Work out the finished part from the listing and answer in its coordinate system (mm). A direction names the side the tool comes from. Round coordinates to 2 decimals unless told otherwise and drop trailing zeros. Order: outer loops, then holes, each group sorted by start corner. A loop starts at its lowest first (then second) coordinate and runs counter-clockwise, first axis right, second up. Notation, with made-up numbers: (33.25, 0.5) - (48.25, 0.5) arc R20 ccw to (48.25, 5.5) - close; hole circle Ø9 at (47, 19.25). An arc over 180 degrees is marked (long way). Answer in a Markdown table with one row per item.
from build123d import *

# Parameters (mm, degrees)
BOSS_EXTRUDE1_DEPTH           = 2
CSK_FOR_M3_SFHCS1_D           = 3
CSK_FOR_M3_SFHCS1_DEPTH       = 9.5
CSK_FOR_M3_SFHCS1_CSINK_D     = 5.6
CSK_FOR_M3_SFHCS1_CSINK_ANGLE = 90
CSK_FOR_M3_SFHCS1_TIP         = 0.901290929
SKETCH6_R                     = 1.05
CUT_EXTRUDE1_DEPTH            = 6
SKETCH7_R                     = 1.05
CUT_EXTRUDE2_DEPTH            = 6
SKETCH8_R                     = 1.05
CUT_EXTRUDE3_DEPTH            = 6
M2_5X0_45_TAPPED_HOLE1_D      = 2.05
M2_5X0_45_TAPPED_HOLE1_DEPTH  = 6.35
M2_5X0_45_TAPPED_HOLE1_TIP    = 0.615882135
TAP_DRILL_FOR_M3X0_5_TAP1_D   = 2.5


with BuildPart() as part:
    # Sketch1 → Boss-Extrude1 (new, symmetric)
    with BuildSketch(Plane(origin=(0, 0, 0), x_dir=(1, 0, 0), z_dir=(0, 1, 0))):
        with BuildLine():
            Line((-48.836461788, 72), (48.836461788, 72))
            ThreePointArc((48.836461788, 72), (0, -87), (-48.836461788, 72))
        make_face()
        with BuildLine():
            Line((-46.314144708, 64), (46.314144708, 64))
            ThreePointArc((46.314144708, 64), (0, -79), (-46.314144708, 64))
        make_face(mode=Mode.SUBTRACT)
    extrude(amount=BOSS_EXTRUDE1_DEPTH, both=True)

    # CSK for M3 SFHCS1
    with Locations(Plane(origin=(-37.681211478, 2, 73.953541508), x_dir=(0, 0, 1), z_dir=(0, 1, 0))):
        with Locations((0, 0), (-141.953541508, -1.578606827), (-141.953541508, 76.941029783), (0, 75.362422956)):
            CounterSinkHole(CSK_FOR_M3_SFHCS1_D / 2, CSK_FOR_M3_SFHCS1_CSINK_D / 2, depth=CSK_FOR_M3_SFHCS1_DEPTH, counter_sink_angle=CSK_FOR_M3_SFHCS1_CSINK_ANGLE)
            with Locations((0, 0, -(CSK_FOR_M3_SFHCS1_DEPTH + CSK_FOR_M3_SFHCS1_TIP / 2))):  # 118° drill point
                Cone(0, CSK_FOR_M3_SFHCS1_D / 2, CSK_FOR_M3_SFHCS1_TIP, mode=Mode.SUBTRACT)

    # Sketch6 → Cut-Extrude1 (cut)
    with BuildSketch(Plane(origin=(75.344210129, 0, -43.5), x_dir=(-0.49999999999999784, 0, -0.86602540378444), z_dir=(0.86602540378444, 0, -0.49999999999999784))):
        Circle(SKETCH6_R)
    cut_extrude1 = extrude(amount=-CUT_EXTRUDE1_DEPTH, mode=Mode.SUBTRACT)

    # Sketch7 → Cut-Extrude2 (cut)
    with BuildSketch(Plane(origin=(75.344210129, 0, 43.5), x_dir=(0.5000000000000047, 0, -0.866025403784436), z_dir=(0.866025403784436, 0, 0.5000000000000047))):
        Circle(SKETCH7_R)
    cut_extrude2 = extrude(amount=-CUT_EXTRUDE2_DEPTH, mode=Mode.SUBTRACT)

    # Mirror1: Cut-Extrude1, Cut-Extrude2 across plane
    add(cut_extrude1.mirror(Plane(origin=(0, 0, 0), x_dir=(0, 0, 1), z_dir=(1, 0, 0))), mode=Mode.SUBTRACT)
    add(cut_extrude2.mirror(Plane(origin=(0, 0, 0), x_dir=(0, 0, 1), z_dir=(1, 0, 0))), mode=Mode.SUBTRACT)

    # Sketch8 → Cut-Extrude3 (cut)
    with BuildSketch(Plane.XY.offset(87)):
        Circle(SKETCH8_R)
    extrude(amount=-CUT_EXTRUDE3_DEPTH, mode=Mode.SUBTRACT)

    # M2.5x0.45 Tapped Hole1
    with Locations(Plane(origin=(33.836461788, 0, -72), x_dir=(-1, 0, 0), z_dir=(0, 0, -1))):
        with Locations((0, 0), (67.672923576, 0)):
            Hole(M2_5X0_45_TAPPED_HOLE1_D / 2, depth=M2_5X0_45_TAPPED_HOLE1_DEPTH)
            with Locations((0, 0, -(M2_5X0_45_TAPPED_HOLE1_DEPTH + M2_5X0_45_TAPPED_HOLE1_TIP / 2))):  # 118° drill point
                Cone(0, M2_5X0_45_TAPPED_HOLE1_D / 2, M2_5X0_45_TAPPED_HOLE1_TIP, mode=Mode.SUBTRACT)

    # Tap Drill for M3x0.5 Tap1 (through all)
    with Locations(Plane(origin=(-83, 2, 0), x_dir=(0, 0, 1), z_dir=(0, 1, 0))):
        with Locations((0, 0), (0, 166)):
            Hole(TAP_DRILL_FOR_M3X0_5_TAP1_D / 2)


solid = part.part
1) The mould has two halves that part along Z. Classify faces 1 (the face through (-73.3, -0.4, 41.2)), 2 (the face through (-1, 0, -72)), 3 (the face through (0, -2, -69)): released by +Z, released by -Z, zero draft, split by the parting line, or undercut.
Filled in:
| item | result |
|---|---|
| face 1 | undercut |
| face 2 | released by -Z |
| face 3 | zero draft |
2) Find section B-B, the plane z = -9.5. Give the vertices of the cut face in (x, y).
Filled in:
| item | result |
|---|---|
| outline | (-86.48, -2) - (-78.43, -2) - (-78.43, 2) - (-86.48, 2) - close; (78.43, -2) - (86.48, -2) - (86.48, 2) - (78.43, 2) - close |
3) Find section A-A, the plane x = -54.5. Give the vertices of the cut face in (y, z), then the cut area to 3 significant figures.
Filled in:
| item | result |
|---|---|
| outline | (-2, -67.81) - (2, -67.81) - (2, -57.19) - (-2, -57.19) - close; (-2, 57.19) - (2, 57.19) - (2, 67.81) - (-2, 67.81) - close |
| area | 85.0 mm^2 |
4) Find the intervals of material crossed by probe 1 along X at (y, z) = (0.05, 0); probe 2 along Z at (x, y) = (-37, -0.4); probe 3 along Y at (x, z) = (0, 85), in increasing order. Write a range as from..to.
Filled in:
| item | result |
|---|---|
| probe 1 | x = -87..-84.25, -81.75..-79, 79..81.75, 84.25..87 |
| probe 2 | z = -72..-64, 69.8..72.62, 75.29..78.74 |
| probe 3 | y = -2..-1.05, 1.05..2 |
5) Each of these flat-tipped pins is pushed along its axis until it touches: pin 1 (12 mm diameter, centred on x = -4.5, z = 71, fed in from +Y); pin 2 (1 mm diameter, centred on x = 0.5, y = 0, fed in from +Z); pin 3 (5 mm diameter, centred on x = -37.68, z = 73.95, fed in from -Y); pin 4 (2 mm diameter, centred on x = 62.5, y = -0.5, fed in from +Z). Where does it stop, or does it pass through?
Filled in:
| item | result |
|---|---|
| pin 1 | passes through |
| pin 2 | stops at z = 81 |
| pin 3 | stops at y = -2 |
| pin 4 | stops at z = 61.54 |
6) Which of the six approach directions +Z, -Z, +X, -X, +Y, -Y give full straight-line access (tool end or side, diameter ignored) to faces 4 (the face through (-1, 0, -64)), 5 (the face through (72.26, 0.05, 42.93))?
Filled in:
| item | result |
|---|---|
| face 4 | +Y, -Y |
| face 5 | none |
